Geometry check sheet. Reference: the model listing, model coordinates, mm. Round coordinates to 2 decimals unless told otherwise and drop trailing zeros. Write each loop counter-clockwise with the first axis right and the second up, starting at its lowest first coordinate (ties: lowest second). Pieces come first, ordered by that corner, then holes. Notation, with made-up numbers: (-30.5, -20) -> (-13.5, -20) arc R7 cw to (-13.5, -8) -> close; hole circle Ø3 at (0.5, -32.75). An arc over 180 degrees is marked (long way). Use a Markdown table: item, result.
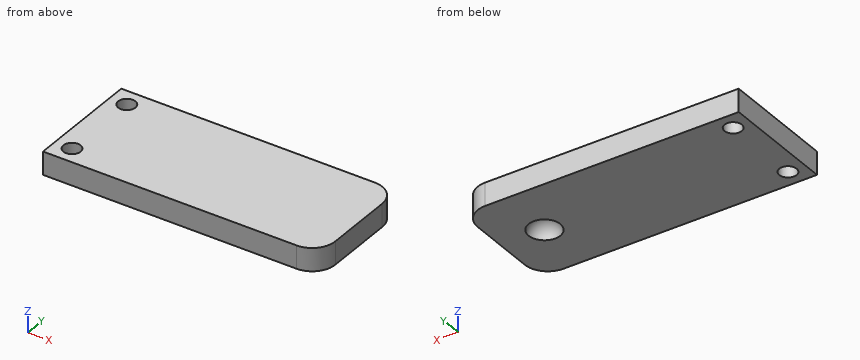
```python
from build123d import *
from build123d.topology import SkipClean

# Parameters (mm, degrees)
SKETCH1_W           = 48
SKETCH1_H           = 20
BOSS_EXTRUDE1_DEPTH = 2
FILLET2_R           = 4
CUT_EXTRUDE1_REACH  = 28.306
SKETCH4_R           = 1.5
CUT_REVOLVE1_ANGLE  = 180


with BuildPart() as part:
    # Sketch1 → Boss-Extrude1 (new, symmetric)
    with BuildSketch(Plane.XY):
        Rectangle(SKETCH1_W, SKETCH1_H)
    extrude(amount=BOSS_EXTRUDE1_DEPTH, both=True)

    # Fillet2
    fillet2_edges = [part.edges().sort_by_distance(p)[0] for p in [
        (24, -10, 0),
        (24, 10, 0),
    ]]
    fillet(fillet2_edges, radius=FILLET2_R)

    # Sketch4 → Cut-Extrude1 (cut, up to next)
    with BuildSketch(Plane(origin=(0, 0, -2), x_dir=(-1, 0, 0), z_dir=(0, 0, -1)), mode=Mode.PRIVATE) as cut_extrude1_sk1:
        with Locations((21, 7)):
            Circle(SKETCH4_R)
    cut_extrude1_tool1 = extrude(cut_extrude1_sk1.sketch, amount=-CUT_EXTRUDE1_REACH, mode=Mode.PRIVATE) & part.part
    # Sketch4 → Cut-Extrude1 (cut, up to next)
    with BuildSketch(Plane(origin=(0, 0, -2), x_dir=(-1, 0, 0), z_dir=(0, 0, -1)), mode=Mode.PRIVATE) as cut_extrude1_sk2:
        with Locations((21, -7)):
            Circle(SKETCH4_R)
    cut_extrude1_tool2 = extrude(cut_extrude1_sk2.sketch, amount=-CUT_EXTRUDE1_REACH, mode=Mode.PRIVATE) & part.part
    add(cut_extrude1_tool1.solids().sort_by_distance((-21, 7, -2))[0], mode=Mode.SUBTRACT)
    add(cut_extrude1_tool2.solids().sort_by_distance((-21, -7, -2))[0], mode=Mode.SUBTRACT)

    # Sketch3 → Cut-Revolve1 (revolve, cut)
    with SkipClean():  # the faces are left unmerged after this step: merging them gives an invalid solid
        with BuildSketch(Plane.XY.offset(-2)):
            with BuildLine():
                ThreePointArc((19.25, 0), (16.5, 2.75), (13.75, 0))
                Line((13.75, 0), (19.25, 0))
            make_face()
            with BuildLine():
                Line((19.25, 0), (13.75, 0))
                ThreePointArc((13.75, 0), (16.5, -2.75), (19.25, 0))
            make_face()
        revolve(axis=Axis((13.75, 0, -2), (1, 0, 0)), revolution_arc=CUT_REVOLVE1_ANGLE, mode=Mode.SUBTRACT)


solid = part.part
```
(1) Section check A-A on x = -21. Record the cut outline in (y, z), plus the area to 3 significant figures.
A:
| item | result |
|---|---|
| outline | (-10, -2) -> (-8.5, -2) -> (-8.5, 2) -> (-10, 2) -> close; (-5.5, -2) -> (5.5, -2) -> (5.5, 2) -> (-5.5, 2) -> close; (8.5, -2) -> (10, -2) -> (10, 2) -> (8.5, 2) -> close |
| area | 56.0 mm2 |
(2) Section check B-B on y = -7.5. Record the cut outline in (x, z).
A:
| item | result |
|---|---|
| outline | (-24, -2) -> (-22.41, -2) -> (-22.41, 2) -> (-24, 2) -> close; (-19.59, -2) -> (23.71, -2) -> (23.71, 2) -> (-19.59, 2) -> close |
(3) Gauge pin test, flat end, axial feed: pin 1 Ø1.8 at (x, y) = (-21, 7) entering from -Z. Record the tip position at first contact, or that the pin passes through.
A:
| item | result |
|---|---|
| pin 1 | passes through |
(4) Thickness scan on line 1 (Y direction, x = -21, z = 0.5); line 2 (Y direction, x = -20, z = 1.85); line 3 (X direction, y = 0, z = -1.6). Record the ranges inside material, lowest first.
A:
| item | result |
|---|---|
| line 1 | y = -10 to -8.5, -5.5 to 5.5, 8.5 to 10 |
| line 2 | y = -10 to -8.12, -5.88 to 5.88, 8.12 to 10 |
| line 3 | x = -24 to 13.78, 19.22 to 24 |
(5) Section check C-C on z = -1.4. Record the cut outline in (x, y).
A:
| item | result |
|---|---|
| outline | (-24, -10) -> (20, -10) arc R4 ccw to (24, -6) -> (24, 6) arc R4 ccw to (20, 10) -> (-24, 10) -> close; hole circle Ø3 at (-21, -7); hole circle Ø3 at (-21, 7); hole circle Ø5.37 at (16.5, 0) |
(6) Section check D-D on y = 6.5. Record the cut outline in (x, z), plus the area to 3 significant figures.
A:
| item | result |
|---|---|
| outline | (-24, -2) -> (-22.41, -2) -> (-22.41, 2) -> (-24, 2) -> close; (-19.59, -2) -> (23.97, -2) -> (23.97, 2) -> (-19.59, 2) -> close |
| area | 181 mm2 |
